Source: CAD feature listing. Evaluate the final solid. Frame: model axes, mm. Face numbers are marked on the shaded views. A direction names the side the tool comes from. Coordinates: 2 decimals unless noted, no trailing zeros. Loops run counter-clockwise (first coordinate to the right, second up) from the corner with the lowest first, then second, coordinate; pieces in that order, holes last. Notation, with made-up numbers: M 20.5,-4 L 53.5,-4 A24 ccw 53.5,14 Z; hole C -6.75,13 d2. An arc over 180 degrees is marked long. One line per question, with ' | ' between items. Start each with the question number.
1. Ray query, probe 1 along X at (y, z) = (1.7, 32.5); probe 2 along Z at (x, y) = (-31, 1.25); probe 3 along X at (y, z) = (3.6, 31.5). Return the intervals inside material, ascending.
2. Section query B-B, the plane x = -80.5. Output: boundary loops of the cut face in (y, z), and give its area (3 significant figures).
3. Pin query (flat end, axial travel): P1, Ø2, axis at x = -59.5, y = 2.5, coming from the +Z side; P2, Ø3, axis at x = -34.5, y = 2.5, coming from the -Z side; P3, Ø25, axis at x = -87.5, z = 23, coming from the -Y side; P4, Ø1.5, axis at y = 3, z = 35, coming from the -X side. Return the tip coordinate at first contact, or that it passes through.
4. Section query D-D, the plane x = -32. Output: boundary loops of the cut face in (y, z).
5. Access query for the marked faces 3 and 4. Directions: +Z, -Z, +X, -X, +Y, -Y. A direction counts if a zero-diameter tool reaches every point of the face in a straight line with its end or side. Return the directions, or none.
6. Section query A-A, the plane y = 1.05. Output: boundary loops of the cut face in (x, z), and give its area (3 significant figures).
7. Mould query, pull axis X, two halves, no side actions, for the marked faces 1 and 2. Classes: pulls with the +X half, pulls with the -X half, needs draft (parallel to the pull), parting line crosses it, or undercut.
8. Section query C-C, the plane z = 37.5. Output: boundary loops of the cut face in (x, y).
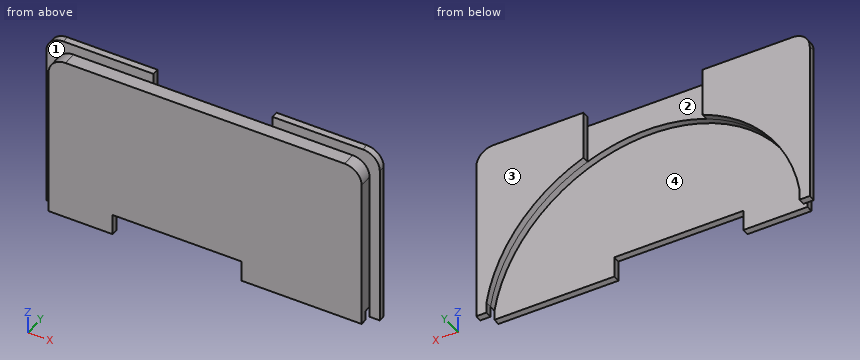
```python
from build123d import *

# Parameters (mm, degrees)
BOSS_EXTRUDE2_DEPTH = 4
CUT_EXTRUDE3_DEPTH  = 4
SKETCH6_R           = 46.644893749
CUT_EXTRUDE4_DEPTH  = 2
SKETCH7_W           = 37.921763703
SKETCH7_H           = 21.966033547
CUT_EXTRUDE5_DEPTH  = 2
CUT_EXTRUDE7_DEPTH  = 10
BOSS_EXTRUDE3_DEPTH = 2


with BuildPart() as part:
    # Sketch4 → Boss-Extrude2 (new body)
    with BuildSketch(Plane(origin=(0, 0, 0), x_dir=(1, 0, 0), z_dir=(0, 1, 0))):
        with BuildLine():
            Line((-107.035735829, 49.14195745), (-15.035735829, 49.14195745))
            Line((-15.035735829, 49.14195745), (-15.035735829, -45.85804255))
            ThreePointArc((-15.035735829, -45.85804255), (-16.500201924, -49.393576456), (-20.035735829, -50.85804255))
            Line((-20.035735829, -50.85804255), (-102.035735829, -50.85804255))
            ThreePointArc((-102.035735829, -50.85804255), (-105.571269735, -49.393576456), (-107.035735829, -45.85804255))
            Line((-107.035735829, -45.85804255), (-107.035735829, 49.14195745))
        make_face()
    extrude(amount=BOSS_EXTRUDE2_DEPTH)

    # Sketch5 → Cut-Extrude3 (cut)
    with BuildSketch(Plane(origin=(0, 4, 0), x_dir=(1, 0, 0), z_dir=(0, 1, 0))):
        with BuildLine():
            Line((-122.184107688, 54.312207558), (-0.881081782, 54.312207558))
            Line((-0.881081782, 54.312207558), (-0.881081782, -1.763818638))
            Line((-0.881081782, -1.763818638), (-15.035735829, -1.763818638))
            ThreePointArc((-15.035735829, -1.763818638), (-61.035735829, 48.088703252), (-107.035735829, -1.763818638))
            Line((-107.035735829, -1.763818638), (-116.20594022, -1.763818638))
            Line((-116.20594022, -1.763818638), (-122.184107688, 54.312207558))
        make_face()
    extrude(amount=-CUT_EXTRUDE3_DEPTH, mode=Mode.SUBTRACT)

    # Sketch6 → Cut-Extrude4 (cut)
    with BuildSketch(Plane(origin=(0, 4, 0), x_dir=(1, 0, 0), z_dir=(0, 1, 0))):
        with Locations((-61.039241489, 3.84195745)):
            Circle(SKETCH6_R)
    extrude(amount=-CUT_EXTRUDE4_DEPTH, mode=Mode.SUBTRACT)

    # Sketch7 → Cut-Extrude5 (cut)
    with BuildSketch(Plane(origin=(0, 2, 0), x_dir=(1, 0, 0), z_dir=(0, 1, 0))):
        with Locations((-69.228954178, 3.760987583)):
            Rectangle(SKETCH7_W, SKETCH7_H)
    extrude(amount=-CUT_EXTRUDE5_DEPTH, mode=Mode.SUBTRACT)

    # Sketch8 → Cut-Extrude7 (cut)
    with BuildSketch(Plane(origin=(0, 2, 0), x_dir=(1, 0, 0), z_dir=(0, 1, 0))):
        Polygon((-107.035735829, 51.823370687), (-12.035735829, 51.823370687), (-15.035735829, -1.011363006), (-107.035735829, -1.011363006), align=None)
    extrude(amount=-CUT_EXTRUDE7_DEPTH, mode=Mode.SUBTRACT)

    # Sketch10 → Boss-Extrude3 (add)
    with BuildSketch(Plane(origin=(0, 4, 0), x_dir=(1, 0, 0), z_dir=(0, 1, 0))):
        with BuildLine():
            Line((-110.035735829, -0.626443871), (-107.035735829, -0.626443871))
            Line((-107.035735829, -0.626443871), (-107.035735829, -3.908437462))
            ThreePointArc((-107.035735829, -3.908437462), (-97.412251623, -25.359930275), (-78.547707812, -39.392284997))
            Line((-78.547707812, -39.392284997), (-78.547707812, -53.939312876))
            Line((-78.547707812, -53.939312876), (-105.035735829, -53.939312876))
            ThreePointArc((-105.035735829, -53.939312876), (-108.571269735, -52.474846782), (-110.035735829, -48.939312876))
            Line((-110.035735829, -48.939312876), (-110.035735829, -0.626443871))
        make_face()
        with BuildLine():
            Line((-12.035735829, -0.626443871), (-12.035735829, -48.939312876))
            ThreePointArc((-12.035735829, -48.939312876), (-13.500201924, -52.474846782), (-17.035735829, -53.939312876))
            Line((-17.035735829, -53.939312876), (-43.530775166, -53.939312876))
            Line((-43.530775166, -53.939312876), (-43.530775166, -39.392284997))
            ThreePointArc((-43.530775166, -39.392284997), (-24.652990845, -25.343430622), (-15.035735829, -3.86671169))
            Line((-15.035735829, -3.86671169), (-15.035735829, -0.626443871))
            Line((-15.035735829, -0.626443871), (-12.035735829, -0.626443871))
        make_face()
    extrude(amount=BOSS_EXTRUDE3_DEPTH)


solid = part.part
```
Taken from the geometry:
1) probe 1: -107.04 to -15.04 | probe 2: 1.01 to 50.86 | probe 3: -107.04 to -91.48, -30.6 to -15.04
2) outline: M 0,7.22 L 2,7.22 L 2,38.55 L 6,38.55 L 6,53.94 L 4,53.94 L 4,50.86 L 0,50.86 Z | area: 143 mm^2
3) P1: z = 50.86 | P2: z = 1.01 | P3: y = 0 | P4: x = -107.04
4) outline: M 0,1.01 L 2,1.01 L 2,32.66 L 6,32.66 L 6,53.94 L 4,53.94 L 4,50.86 L 0,50.86 Z
5) face 3: +Z, -Z, +X, -X, +Y | face 4: -Z, +Y
6) outline: M -107.04,1.01 L -88.19,1.01 L -88.19,7.22 L -50.27,7.22 L -50.27,1.01 L -15.04,1.01 L -15.04,45.86 A5 ccw -20.04,50.86 L -102.04,50.86 A5 ccw -107.04,45.86 Z | area: 4,340 mm^2
7) face 1: needs draft | face 2: undercut
8) outline: M -110.04,4 L -107.04,4 L -107.04,0 L -15.04,0 L -15.04,4 L -12.04,4 L -12.04,6 L -39.44,6 L -39.44,2 L -82.64,2 L -82.64,6 L -110.04,6 Z
